For this review, take the finished solid that the model builds, in its own axes (mm). Coordinates: 2 decimals unless noted, no trailing zeros. Write each loop counter-clockwise with the first axis right and the second up, starting at its lowest first coordinate (ties: lowest second). Pieces come first, ordered by that corner, then holes. Notation, with made-up numbers: (-1, 34) - (6, 34) arc R9 cw to (6, 44) - close; hole circle Ø8 at (52, 63). An arc over 180 degrees is marked (long way). Use one line per item in the form item = value. Start each with the question number.
1) For L1, parallel to X at y = 0, z = 1.95; L2, parallel to Y at x = 42.5, z = 1.05 (3 decimals); L3, parallel to Y at x = -8, z = 1, list the stretches that pass through material, from the lowest coordinate up. Write a range as from..to.
2) We need section A-A (x = 35). Give the boundary of the cut face in (y, z), plus the area to 3 significant figures.
3) We need section C-C (x = -42). Give the boundary of the cut face in (y, z).
4) We need section B-B (y = 18). Give the boundary of the cut face in (x, z).
5) We need section D-D (z = 0.9). Count the separate pieces of the cut face and the enclosed holes in it, plus the area to 3 significant figures.
6) Insertion check: P1, Ø2.5, axis at x = 18, y = 18, coming from the +Z side (3 decimals); P2, Ø1.5, axis at x = -2, z = 1.5, coming from the +Y side. Each pin has a flat end and moves straight along its axis. Give the tip position at first contact, or say it passes through.
```python
from build123d import *

# Parameters (mm, degrees)
SKETCH_1_W          = 103
SKETCH_1_H          = 67.45
EXTRUDE_1_DEPTH     = 3
SKETCH_2_R          = 1.5
SKETCH_2_R_2        = 1.55
CUT_EXTRUDE_1_DEPTH = 10
CUT_EXTRUDE_2_DEPTH = 10
FILLET_2_R          = 2.5


with BuildPart() as part:
    # 草图1 → 凸台-拉伸1 (new body)
    with BuildSketch(Plane.XY):
        Rectangle(SKETCH_1_W, SKETCH_1_H)
    extrude(amount=EXTRUDE_1_DEPTH)

    # 草图2 → 切除-拉伸1 (cut)
    with BuildSketch(Plane.XY.offset(3)):
        with Locations((-18, 18)):
            Circle(SKETCH_2_R)
        with Locations((18, 18)):
            Circle(SKETCH_2_R)
        with Locations((18, -18)):
            Circle(SKETCH_2_R)
        with Locations((-18, -18)):
            Circle(SKETCH_2_R)
        with Locations((-42.499997562, 28.725)):
            Circle(SKETCH_2_R_2)
        with Locations((-42.499997562, -28.725)):
            Circle(SKETCH_2_R_2)
        with Locations((42.5, -28.725)):
            Circle(SKETCH_2_R_2)
        with Locations((42.5, 28.725)):
            Circle(SKETCH_2_R_2)
    extrude(amount=-CUT_EXTRUDE_1_DEPTH, mode=Mode.SUBTRACT)

    # 草图3 → 切除-拉伸2 (cut)
    with BuildSketch(Plane.XY.offset(3)):
        Polygon((-39.499997562, 24.136880962), (-39.499997562, -24.136880962), (-21, -16.038411836), (-21, 16.038411836), align=None)
        Polygon((-17.162839154, 22), (-23.38778026, 24.725), (-43.947218774, 33.725), (43.947221211, 33.725), (23.387782698, 24.725), (17.162841592, 22), align=None)
        Polygon((39.5, 24.136880962), (21, 16.038410769), (21, -16.038411758), (39.5, -24.136881145), align=None)
        Polygon((-23.38778026, -24.725), (-17.162839154, -22), (17.162839231, -22), (23.387780956, -24.725), (43.947221515, -33.725), (-43.947218774, -33.725), align=None)
        Polygon((-2.828427125, 0), (-16, 13.171572875), (-16, -13.171572875), align=None)
        Polygon((13.171572875, 16), (-13.171572875, 16), (0, 2.828427125), align=None)
        Polygon((2.828427125, 0), (16, 13.171572875), (16, -13.171572875), align=None)
        Polygon((-13.171572875, -16), (0, -2.828427125), (13.171572875, -16), align=None)
    extrude(amount=-CUT_EXTRUDE_2_DEPTH, mode=Mode.SUBTRACT)

    # 圆角2
    fillet_2_edges = [part.edges().sort_by_distance(p)[0] for p in [
        (17.162841592, 22, 1.5),
        (-17.162839154, 22, 1.5),
        (-43.947218774, 33.725, 1.5),
        (43.947221211, 33.725, 1.5),
        (39.5, 24.136880962, 1.5),
        (39.5, -24.136881145, 1.5),
        (21, -16.038411758, 1.5),
        (21, 16.038410769, 1.5),
        (13.171572875, -16, 1.5),
        (-13.171572875, -16, 1.5),
        (0, -2.828427125, 1.5),
        (13.171572875, 16, 1.5),
        (0, 2.828427125, 1.5),
        (-13.171572875, 16, 1.5),
        (16, -13.171572875, 1.5),
        (2.828427125, 0, 1.5),
        (16, 13.171572875, 1.5),
        (-39.499997562, 24.136880962, 1.5),
        (-21, 16.038411836, 1.5),
        (-21, -16.038411836, 1.5),
        (-39.499997562, -24.136880962, 1.5),
        (-51.5, 33.725, 1.5),
        (51.5, 33.725, 1.5),
        (51.5, -33.725, 1.5),
        (-51.5, -33.725, 1.5),
        (-2.828427125, 0, 1.5),
        (-16, -13.171572875, 1.5),
        (-16, 13.171572875, 1.5),
        (-43.947218774, -33.725, 1.5),
        (-17.162839154, -22, 1.5),
        (17.162839231, -22, 1.5),
        (43.947221515, -33.725, 1.5),
    ]]
    fillet(fillet_2_edges, radius=FILLET_2_R)


solid = part.part
```
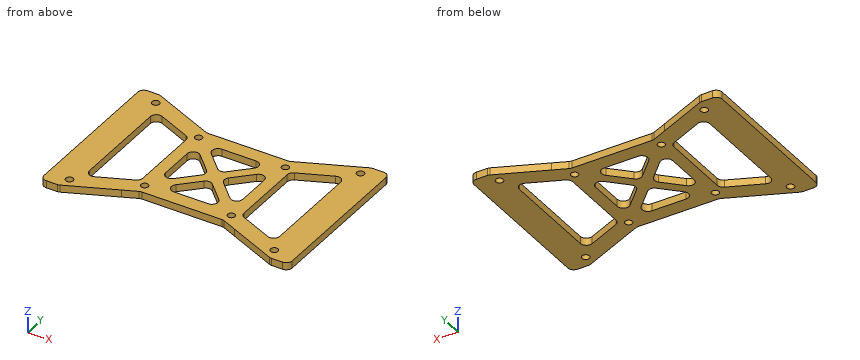
Determined:
q1.L1 = -51.5..-39.5, -21..-16, -3.86..3.86, 16..21, 39.5..51.5
q1.L2 = -33.091..-30.275, -27.175..27.175, 30.275..33.091
q1.L3 = -22..-15.85, -10.83..-5.17, 5.17..10.83, 15.85..22
q2.outline = (-29.81, 0) - (-22.17, 0) - (-22.17, 3) - (-29.81, 3) - close; (22.17, 0) - (29.81, 0) - (29.81, 3) - (22.17, 3) - close
q2.area = 45.8 mm²
q3.outline = (-32.87, 0) - (-30.19, 0) - (-30.19, 3) - (-32.87, 3) - close; (-27.26, 0) - (27.26, 0) - (27.26, 3) - (-27.26, 3) - close; (30.19, 0) - (32.87, 0) - (32.87, 3) - (30.19, 3) - close
q4.outline = (-51.5, 0) - (-39.5, 0) - (-39.5, 3) - (-51.5, 3) - close; (-25.48, 0) - (-19.5, 0) - (-19.5, 3) - (-25.48, 3) - close; (-16.5, 0) - (16.5, 0) - (16.5, 3) - (-16.5, 3) - close; (19.5, 0) - (25.48, 0) - (25.48, 3) - (19.5, 3) - close; (39.5, 0) - (51.5, 0) - (51.5, 3) - (39.5, 3) - close
q5.separate_pieces = 1
q5.enclosed_holes = 14
q5.area = 3,350 mm²
q6.P1 = through
q6.P2 = 22
